CAD build for the part. Positions are in the model's coordinates, mm. Coordinates: 2 decimals unless noted, no trailing zeros. Write each loop counter-clockwise with the first axis right and the second up, starting at its lowest first coordinate (ties: lowest second). Pieces come first, ordered by that corner, then holes. Notation, with made-up numbers: (84, 10.5) -> (136, 10.5) arc R26 ccw to (136, 26.5) -> close; hole circle Ø6 at (-10, 89). An arc over 180 degrees is marked (long way). Answer as CSV lines item,"result". Start each with the question number.
```python
from build123d import *

# Parameters (mm, degrees)
SKETCH1_R           = 50
BOSS_EXTRUDE1_DEPTH = 200
CHAMFER1_SIZE       = 40
FILLET1_R           = 12
FILLET2_R           = 12
CHAMFER2_SIZE       = 10


with BuildPart() as part:
    # Sketch1 → Boss-Extrude1 (new body, symmetric)
    with BuildSketch(Plane(origin=(0, 0, 0), x_dir=(0, 0, -1), z_dir=(1, 0, 0))):
        Circle(SKETCH1_R)
    extrude(amount=BOSS_EXTRUDE1_DEPTH, both=True)

    # Chamfer1
    chamfer1_edges = [part.edges().sort_by_distance(p)[0] for p in [
        (200, 0, 50),
    ]]
    chamfer(chamfer1_edges, length=CHAMFER1_SIZE)

    # Fillet1
    fillet1_edges = [part.edges().sort_by_distance(p)[0] for p in [
        (200, 0, 10),
    ]]
    fillet(fillet1_edges, radius=FILLET1_R)

    # Fillet2
    fillet2_edges = [part.edges().sort_by_distance(p)[0] for p in [
        (160, 0, 50),
    ]]
    fillet(fillet2_edges, radius=FILLET2_R)

    # Chamfer2
    chamfer2_edges = [part.edges().sort_by_distance(p)[0] for p in [
        (-200, 0, 50),
    ]]
    chamfer(chamfer2_edges, length=CHAMFER2_SIZE)


solid = part.part
```
1. Wall check: line 1 (Z direction, x = 135.5, y = -30); line 2 (X direction, y = -4, z = -4.5); line 3 (Z direction, x = -159.5, y = 25). Give the ranges that are in metal, low to high.
2. Flat gauge pins, fed straight in: P1, Ø4, axis at y = -4, z = 14.5, coming from the +X side; P2, Ø5, axis at x = 150, z = -5, coming from the +Y side; P3, Ø10, axis at y = -35.5, z = 30.5, coming from the -X side. Where does each tip first touch, or does it go through?
3. Cut at A-A (x = 59.5). Give the cut face in (y, z), then the cut area to 3 significant figures.
Geometry check:
1,line 1,"-40 to 40"
1,line 2,"-200 to 199.96"
1,line 3,"-43.3 to 43.3"
2,P1,"x = 196.93"
2,P2,"y = 49.94"
2,P3,"x = -198.2"
3,outline,"circle Ø100 at (0, 0)"
3,area,"7,850 mm²"
